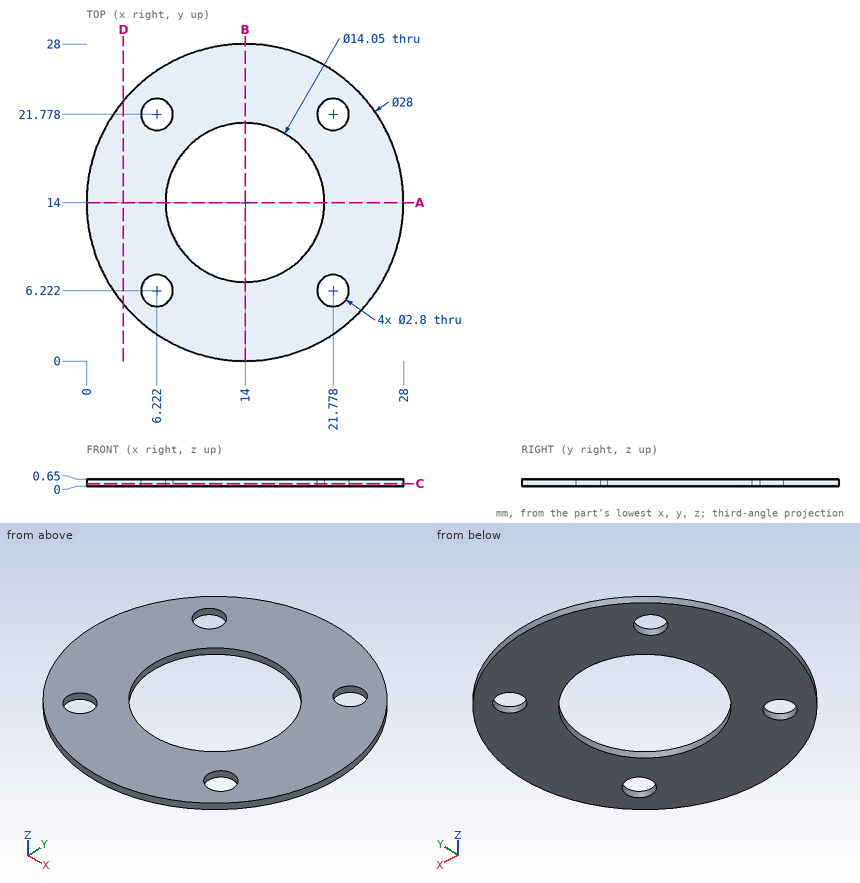
The drawing under review shows one solid part. Ordinate dimensions are in mm from its lowest x, y, z. Round coordinates to 2 decimals unless told otherwise and drop trailing zeros. Loops run counter-clockwise (first coordinate to the right, second up) from the corner with the lowest first, then second, coordinate; pieces in that order, holes last. Notation, with made-up numbers: (61, 73.25) - (84, 73.25) arc R35 cw to (84, 111.25) - close; hole circle Ø1 at (35.5, -36.75). An arc over 180 degrees is marked (long way). One line per item, written item: value. Start each with the question number.
1) Consider section D-D on x = 3.25. Give the boundary of the cut face in (y, z).
2) To check wall thickness, follow L1, parallel to Y at x = 14, z = 0.55 (3 decimals); L2, parallel to X at y = 22.25, z = 0.1; L3, parallel to X at y = 13.75, z = 0.55. State the ranges of each line that lie inside material, in increasing order. Write a range as from..to.
3) Consider section A-A on y = 14. Give the boundary of the cut face in (x, z) (3 decimals).
4) Consider section C-C on z = 0.25. Give the number of separate pieces and of enclosed holes in the cut face, then the cut area to 3 significant figures.
Reported:
1. outline: (5.03, 0) - (22.97, 0) - (22.97, 0.65) - (5.03, 0.65) - close
2. L1: y = 0..6.975, 21.025..28
2. L2: x = 2.69..4.9, 7.54..20.46, 23.1..25.31
2. L3: x = 0..6.98, 21.02..28
3. outline: (0, 0) - (6.975, 0) - (6.975, 0.65) - (0, 0.65) - close; (21.025, 0) - (28, 0) - (28, 0.65) - (21.025, 0.65) - close
4. separate pieces: 1
4. enclosed holes: 5
4. area: 436 mm^2
